Autodesk Inventor part; units mm, degrees
ref_plane "YZ Plane" through (0, 0, 0) normal (1, 0, 0) x (0, 1, 0)
ref_plane "XZ Plane" through (0, 0, 0) normal (0, 1, 0) x (-1, 0, 0)
ref_plane "XY Plane" through (0, 0, 0) normal (0, 0, 1) x (1, 0, 0)
sketch "Sketch1" plane through (0, 0, 0) normal (0, 1, 0) x (-1, 0, 0)
  line L0 (-25, 42.5) -> (25, 42.5)
  line L1 (28, 39.5) -> (28, -40.5)
  line L2 (26, -42.5) -> (-25, -42.5)
  line L3 (-28, -39.5) -> (-28, 39.5)
  line L4 (-28, 42.5) -> (28, -42.5) construction
  line L5 (28, 42.5) -> (-28, -42.5) construction
  arc A0 (26, -42.5) -> (28, -40.5) centre (26, -40.5) ccw
  arc A1 (-28, -39.5) -> (-25, -42.5) centre (-25, -39.5) ccw
  arc A2 (-25, 42.5) -> (-28, 39.5) centre (-25, 39.5) ccw
  arc A3 (28, 39.5) -> (25, 42.5) centre (25, 39.5) ccw
  line L6 (30, -40.5) -> (30, 39.5)
  arc A4 (30, 39.5) -> (25, 44.5) centre (25, 39.5) ccw
  line L7 (25, 44.5) -> (-25, 44.5)
  arc A5 (-25, 44.5) -> (-30, 39.5) centre (-25, 39.5) ccw
  line L8 (-30, 39.5) -> (-30, -39.5)
  arc A6 (-30, -39.5) -> (-25, -44.5) centre (-25, -39.5) ccw
  line L9 (-25, -44.5) -> (26, -44.5)
  arc A7 (26, -44.5) -> (30, -40.5) centre (26, -40.5) ccw
  point P0 (0, 0)
  dimension "d0" = 56
  dimension "d1" = 85
  dimension "d2" = 2
  dimension "d3" = 3
  dimension "d4" = 2
extrude "Extrusion1" add sketch "Sketch1" along normal blind 1
sketch "Sketch2" plane through (0, 0, 0) normal (0, -1, 0) x (1, 0, 0)
  arc A0 (-25, 44.5) -> (-30, 39.5) centre (-25, 39.5) ccw
  line L0 (-25, 44.5) -> (25, 44.5)
  arc A1 (30, 39.5) -> (25, 44.5) centre (25, 39.5) ccw
  line L1 (30, 39.5) -> (30, -39.5)
  arc A2 (25, -44.5) -> (30, -39.5) centre (25, -39.5) ccw
  line L2 (25, -44.5) -> (-26, -44.5)
  arc A3 (-30, -40.5) -> (-26, -44.5) centre (-26, -40.5) ccw
  line L3 (-30, -40.5) -> (-30, 39.5)
  line L4 (-26, -44.5) -> (25, -44.5)
  line L5 (30, -39.5) -> (30, 39.5)
  line L6 (25, 44.5) -> (-25, 44.5)
  line L7 (-30, 39.5) -> (-30, -40.5)
  line L8 (-30, -44.5) -> (30, 44.5) construction
  line L9 (30, -44.5) -> (-30, 44.5) construction
  arc A4 (-25, 44.5) -> (-30, 39.5) centre (-25, 39.5) ccw
  arc A5 (30, 39.5) -> (25, 44.5) centre (25, 39.5) ccw
  arc A6 (25, -42.5) -> (28, -39.5) centre (25, -39.5) ccw
  arc A7 (25, -44.5) -> (30, -39.5) centre (25, -39.5) ccw
  arc A8 (-30, -40.5) -> (-26, -44.5) centre (-26, -40.5) ccw
  line L10 (25, 40.5) -> (-25, 40.5)
  arc A9 (-25, 40.5) -> (-26, 39.5) centre (-25, 39.5) ccw
  line L11 (-26, 39.5) -> (-26, -40.5)
  line L12 (-26, -40.5) -> (25, -40.5)
  arc A10 (25, -40.5) -> (26, -39.5) centre (25, -39.5) ccw
  line L13 (26, -39.5) -> (26, 39.5)
  arc A11 (26, 39.5) -> (25, 40.5) centre (25, 39.5) ccw
  point P0 (0, 0)
  point P1 (-26, -40.5)
  dimension "d12" = 4
extrude "Extrusion2" add sketch "Sketch2" along normal blind 2.5
sketch "Sketch3" plane through (25, 1, -44.5) normal (0, 0, -1) x (-1, 0, 0)
  line L0 (51, -3.5) -> (51, 0)
  line L1 (51, 0) -> (0, 0)
  line L2 (0, 0) -> (0, 1.5)
  line L3 (0, 1.5) -> (51, 1.5)
  line L4 (51, 1.5) -> (51, 0)
  point P0 (25, -1)
  dimension "d9" = 1.5
extrude "Extrusion3" add sketch "Sketch3" against normal blind 4
sketch "Sketch4" plane through (0, -2.5, 0) normal (0, -1, 0) x (1, 0, 0)
  line L0 (25, 44.5) -> (-25, 44.5)
  line L1 (-30, 39.5) -> (-30, -40.5)
  line L2 (-26, -44.5) -> (25, -44.5)
  line L3 (30, -39.5) -> (30, 39.5)
  line L4 (30, 44.5) -> (-30, -44.5) construction
  line L5 (-30, 44.5) -> (30, -44.5) construction
  line L6 (-26, -44.5) -> (25, -44.5)
  line L7 (-30, 39.5) -> (-30, -40.5)
  arc A0 (25, -44.5) -> (30, -39.5) centre (25, -39.5) ccw
  arc A1 (-30, -40.5) -> (-26, -44.5) centre (-26, -40.5) ccw
  arc A2 (-25, 44.5) -> (-30, 39.5) centre (-25, 39.5) ccw
  arc A3 (30, 39.5) -> (25, 44.5) centre (25, 39.5) ccw
  arc A4 (25, -44.5) -> (30, -39.5) centre (25, -39.5) ccw
  line L8 (25, -40.5) -> (-26, -40.5)
  arc A5 (-30, -40.5) -> (-26, -44.5) centre (-26, -40.5) ccw
  arc A6 (-25, 44.5) -> (-30, 39.5) centre (-25, 39.5) ccw
  arc A7 (30, 39.5) -> (25, 44.5) centre (25, 39.5) ccw
  line L9 (25, 44.5) -> (-25, 44.5)
  point P0 (0, 0)
extrude "Extrusion4" add sketch "Sketch4" along normal blind 1
sketch "Sketch5" plane through (25, 2.5, -44.5) normal (0, 0, -1) x (-1, 0, 0)
  line L0 (51, -6) -> (0, -6)
  line L1 (18, -5) -> (32, -5)
  line L2 (32, -5) -> (32, -2.5)
  line L3 (32, -2.5) -> (18, -2.5)
  line L4 (18, -2.5) -> (18, -5)
  line L5 (18, -5) -> (32, -2.5) construction
  line L6 (32, -5) -> (18, -2.5) construction
  point P0 (25, -2.5)
  point P1 (25, -3.75)
  dimension "d16" = 14
  dimension "d17" = 1
  dimension "d18" = 2.5
extrude "Extrusion5" cut sketch "Sketch5" against normal up to surface (4 mm away)
properties part number "piholder-v1"
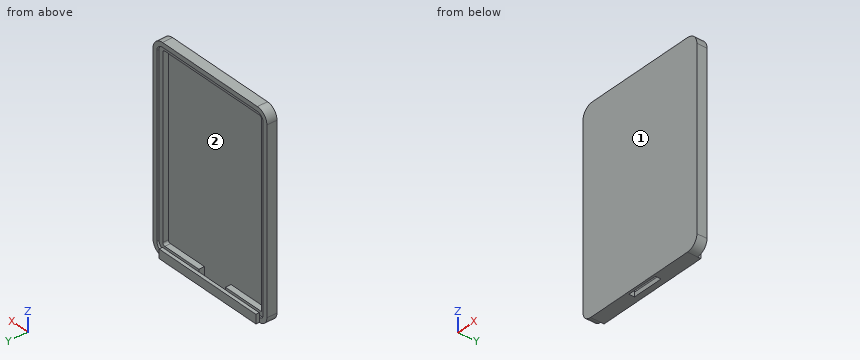
Geometry check sheet. Reference: the model listing, model coordinates, mm. Face numbers are marked on the shaded views. Coordinates: 2 decimals unless noted, no trailing zeros. Order: outer loops, then holes, each group sorted by start corner. A loop starts at its lowest first (then second) coordinate and runs counter-clockwise, first axis right, second up.
Q1. Depth check by flat-ended pin: pin 1 Ø8 at (x, z) = (-8, -26.5) entering from +Y; pin 2 Ø3 at (y, z) = (-1, -43) entering from +X; pin 3 Ø2 at (y, z) = (-2, -42.5) entering from -X. Enter the tip coordinate at first touch or a pass-through.
Reply:
pin 1: stops at y = -2.5
pin 2: stops at x = 29.58
pin 3: stops at x = -29.87
Q2. Sectioned sample at B-B on z = -36. Record the cut outline in (x, y), and give its area (3 significant figures).
Reply:
outline: (-30, -3.5) - (30, -3.5) - (30, 1) - (28, 1) - (28, 0) - (26, 0) - (26, -2.5) - (-26, -2.5) - (-26, 0) - (-28, 0) - (-28, 1) - (-30, 1) - close
area: 84.0 mm2
Q3. Sectioned sample at C-C on x = 22. Record the cut outline in (y, z), and give its area (3 significant figures).
Reply:
outline: (-3.5, -44.5) - (2.5, -44.5) - (2.5, -40.5) - (1, -40.5) - (1, -42.5) - (0, -42.5) - (0, -40.5) - (-2.5, -40.5) - (-2.5, 40.5) - (0, 40.5) - (0, 42.5) - (1, 42.5) - (1, 44.5) - (-3.5, 44.5) - close
area: 119 mm2
Q4. Sectioned sample at A-A on x = -6. Record the cut outline in (y, z).
Reply:
outline: (-3.5, -44.5) - (-2.5, -44.5) - (-2.5, 40.5) - (0, 40.5) - (0, 42.5) - (1, 42.5) - (1, 44.5) - (-3.5, 44.5) - close; (0, -44.5) - (2.5, -44.5) - (2.5, -40.5) - (1, -40.5) - (1, -42.5) - (0, -42.5) - close
Q5. Draft check along X on the marked faces 1 and 2. Enter one of: released by +X, released by -X, zero draft, split by the parting line, or undercut.
Reply:
face 1: zero draft
face 2: undercut
Q6. Thickness scan on probe 1 along X at (y, z) = (-0.8, 10); probe 2 along Z at (x, y) = (14, -1.1); probe 3 along X at (y, z) = (0.8, 37.5). Record the ranges inside material, lowest first.
Reply:
probe 1: x = -30 to -26, 26 to 30
probe 2: z = -44.5 to -40.5, 40.5 to 44.5
probe 3: x = -30 to -28, 28 to 30
